Read the model definition and answer for the solid it produces. Units are mm, in the model's axes. Face numbers are marked on the shaded views. A direction names the side the tool comes from. Coordinates: 2 decimals unless noted, no trailing zeros. Loops run counter-clockwise (first coordinate to the right, second up) from the corner with the lowest first, then second, coordinate; pieces in that order, holes last. Notation, with made-up numbers: (12, 9) -> (61, 9) arc R18 ccw to (61, 37) -> close; hole circle Ø10 at (74, 39). An arc over 180 degrees is marked (long way). Answer as a JSON object with one key per item and string values. Group by question number.
Q1. Straight lines are drawn through the part: line 1 along Z through (x, y) = (0.5, 0.5); line 2 along Y through (x, z) = (0.5, 19); line 3 along X through (y, z) = (-1, 6). For each, find the intervals that lie inside material, in ascending order. Write a range as [from, to].
Q2. The part is cut by section A-A on x = 0. Write down the section's boundary in (y, z).
Q3. Each of these flat-tipped pins is pushed along its axis until it touches: P1, Ø5, axis at x = 3.5, z = 4, coming from the +Y side; P2, Ø3, axis at x = 3, z = 3.5, coming from the +Y side; P3, Ø1, axis at x = -1, z = 13.5, coming from the -Y side. Where does it stop, or does it pass through?
Q4. Determine the mould class of the marked faces 1, 2, 3 and 4 for opening direction X: released by +X, released by -X, zero draft, split by the parting line, or undercut.
Q5. For the marked faces 5 and 6, determine the directions among +Z, -Z, +X, -X, +Y, -Y from which every point of the face is accessible in a straight line to the end or side of a thin tool.
Q6. The part is cut by section B-B on z = 16.5. Write down the section's boundary in (x, y), and give its area (3 significant figures).
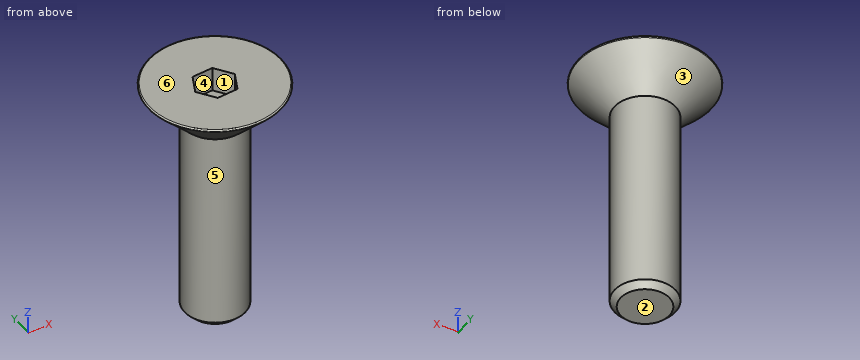
Autodesk Inventor part; units mm, degrees
ref_plane "YZ Plane" through (0, 0, 0) normal (1, 0, 0) x (0, 1, 0)
ref_plane "XZ Plane" through (0, 0, 0) normal (0, 1, 0) x (-1, 0, 0)
ref_plane "XY Plane" through (0, 0, 0) normal (0, 0, 1) x (1, 0, 0)
sketch "Sketch1" plane through (0, 0, 0) normal (0, 0, 1) x (1, 0, 0)
  circle A0 centre (0, 0) radius 2.5
  dimension "Diameter" = 5
extrude "Extrusion1" add sketch "Sketch1" along normal blind 16.9
sketch "Sketch2" plane through (0, 0, 16.9) normal (0, 0, 1) x (1, 0, 0)
  circle A0 centre (0, 0) radius 2.5
extrude "Extrusion2" add sketch "Sketch2" along normal blind 3.1 draft 45
sketch "Sketch3" plane through (0, 0, 20) normal (0, 0, 1) x (1, 0, 0)
  circle A0 centre (0, 0) radius 5.6
  circle A1 centre (0, 0) radius 1.7321 construction
  line L0 (0.725, 1.573) -> (1.7248, 0.1586)
  line L1 (1.7248, 0.1586) -> (0.9997, -1.4144)
  line L2 (0.9997, -1.4144) -> (-0.725, -1.573)
  line L3 (-0.725, -1.573) -> (-1.7248, -0.1586)
  line L4 (-1.7248, -0.1586) -> (-0.9997, 1.4144)
  line L5 (-0.9997, 1.4144) -> (0.725, 1.573)
  dimension "Hex_Width" = 3
extrude "Extrusion3" cut sketch "Sketch3" against normal blind 2 contours L0 L1 L2 L3 L4 L5
thread "Thread1"
chamfer "Chamfer2" distance 0.5 angle 45 1 edges at (-2.5, 0, 0)
fillet "Fillet1" radius 0.1 1 edges at (-5.6, 0, 20)
equation "\"d10\" = Thread_Length"
equation "\"d13\" = Chamfer"
equation "\"Thread_Length\" = 16.9"
properties part number "SCREW, FLAT HD, P, 5, M5X0_8X20MM"
Final values:
{
 "1": {"line 1": "z = [0, 18]", "line 2": "y = [-4.57, -1.46], [1.55, 4.57]", "line 3": "x = [-2.29, 2.29]"},
 "2": {"outline": "(-5.43, 19.83) -> (-2.5, 16.9) -> (-2.5, 0.5) -> (-2, 0) -> (2, 0) -> (2.5, 0.5) -> (2.5, 16.9) -> (5.43, 19.83) arc R0.1 ccw to (5.36, 20) -> (1.51, 20) -> (1.51, 18) -> (-1.51, 18) -> (-1.51, 20) -> (-5.36, 20) arc R0.1 ccw to start"},
 "3": {"P1": "stops at y = 2.29", "P2": "stops at y = 2", "P3": "stops at y = -2.45"},
 "4": {"face 1": "undercut", "face 2": "zero draft", "face 3": "split by the parting line", "face 4": "undercut"},
 "5": {"face 5": "-Z", "face 6": "+Z, +X, -X, +Y, -Y"},
 "6": {"outline": "circle Ø5 at (0, 0)", "area": "19.6 mm2"}
}
